```python
from build123d import *

# Parameters (mm, degrees)
CROQUIS1_W              = 240
CROQUIS1_H              = 70
SALIENTE_EXTRUIR1_DEPTH = 5
CROQUIS2_R              = 2.25
CORTAR_EXTRUIR1_DEPTH   = 126.39936204
CROQUIS5_W              = 35
CROQUIS5_H              = 10
CORTAR_EXTRUIR4_DEPTH   = 126.39936204
CROQUIS6_R              = 2.5
CORTAR_EXTRUIR5_DEPTH   = 126.39936204


with BuildPart() as part:
    # Croquis1 → Saliente-Extruir1 (new, symmetric)
    with BuildSketch(Plane(origin=(0, 0, 0), x_dir=(1, 0, 0), z_dir=(0, 1, 0))):
        Rectangle(CROQUIS1_W, CROQUIS1_H)
    extrude(amount=SALIENTE_EXTRUIR1_DEPTH, both=True)

    # Croquis2 → Cortar-Extruir1 (cut, through all)
    with BuildSketch(Plane(origin=(0, 5, 0), x_dir=(1, 0, 0), z_dir=(0, 1, 0))):
        with Locations(Location((-115, 20, 0), (0, 0, 270))):
            Circle(CROQUIS2_R)
        with Locations(Location((-115, -20, 0), (0, 0, 270))):
            Circle(CROQUIS2_R)
        with Locations(Location((115, -20, 0), (0, 0, 90))):
            Circle(CROQUIS2_R)
        with Locations(Location((115, 20, 0), (0, 0, 90))):
            Circle(CROQUIS2_R)
    extrude(amount=-CORTAR_EXTRUIR1_DEPTH, mode=Mode.SUBTRACT)

    # Croquis5 → Cortar-Extruir4 (cut, through all)
    with BuildSketch(Plane(origin=(0, 5, 0), x_dir=(1, 0, 0), z_dir=(0, 1, 0))):
        with Locations((-31.75, 21.46)):
            Rectangle(CROQUIS5_W, CROQUIS5_H)
        with Locations((-31.75, -21.71)):
            Rectangle(CROQUIS5_W, CROQUIS5_H)
        with Locations((31.75, 21.46)):
            Rectangle(CROQUIS5_W, CROQUIS5_H)
        with Locations((31.75, -21.71)):
            Rectangle(CROQUIS5_W, CROQUIS5_H)
    extrude(amount=-CORTAR_EXTRUIR4_DEPTH, mode=Mode.SUBTRACT)

    # Croquis6 → Cortar-Extruir5 (cut, through all)
    with BuildSketch(Plane(origin=(0, 5, 0), x_dir=(1, 0, 0), z_dir=(0, 1, 0))):
        with Locations(Location((71.38, 0, 0), (0, 0, 270))):
            Circle(CROQUIS6_R)
        with Locations(Location((-91.85, 0, 0), (0, 0, 270))):
            Circle(CROQUIS6_R)
    extrude(amount=-CORTAR_EXTRUIR5_DEPTH, mode=Mode.SUBTRACT)


solid = part.part
```
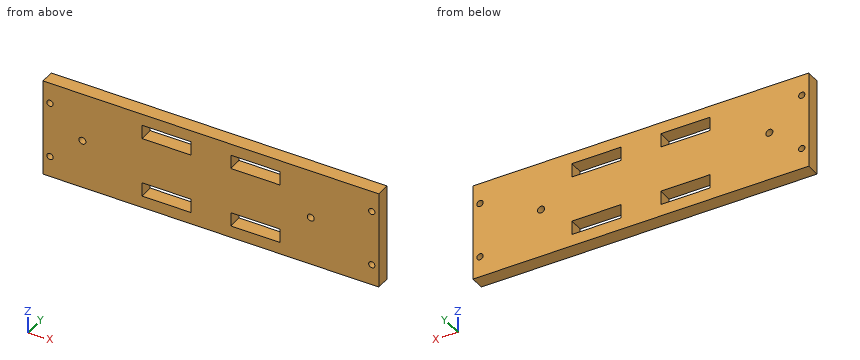
Here's how the part is built. I have some questions about the finished solid (model axes, mm). Coordinates: 2 decimals unless noted, no trailing zeros. Order: outer loops, then holes, each group sorted by start corner. A loop starts at its lowest first (then second) coordinate and runs counter-clockwise, first axis right, second up.
1) Imagine slicing it at B-B on z = 20. List the corners of the cut face in (x, y) for me, and give its area (3 significant figures).
2) Imagine slicing it at C-C on y = -2.5. State how many separate pieces and enclosed holes the cut face has, and give its area (3 significant figures).
3) Imagine slicing it at D-D on x = -91.85. List the corners of the cut face in (y, z) for me, and give its area (3 significant figures).
4) I need wall thicknesses on line 1 (X direction, y = -1, z = 20); line 2 (X direction, y = -1.25, z = 23.5); line 3 (Z direction, x = 115, y = 1). Which ranges of each line are inside material? Lowest first, please.
5) Imagine slicing it at A-A on x = 42. List the corners of the cut face in (y, z) for me.
Response values:
1. outline: (-120, -5) - (-117.25, -5) - (-117.25, 5) - (-120, 5) - close; (-112.75, -5) - (-49.25, -5) - (-49.25, 5) - (-112.75, 5) - close; (-14.25, -5) - (14.25, -5) - (14.25, 5) - (-14.25, 5) - close; (49.25, -5) - (112.75, -5) - (112.75, 5) - (49.25, 5) - close; (117.25, -5) - (120, -5) - (120, 5) - (117.25, 5) - close
1. area: 1,610 mm2
2. separate pieces: 1
2. enclosed holes: 10
2. area: 15,300 mm2
3. outline: (-5, -35) - (5, -35) - (5, -2.5) - (-5, -2.5) - close; (-5, 2.5) - (5, 2.5) - (5, 35) - (-5, 35) - close
3. area: 650 mm2
4. line 1: x = -120 to -117.25, -112.75 to -49.25, -14.25 to 14.25, 49.25 to 112.75, 117.25 to 120
4. line 2: x = -120 to -49.25, -14.25 to 14.25, 49.25 to 120
4. line 3: z = -35 to -22.25, -17.75 to 17.75, 22.25 to 35
5. outline: (-5, -35) - (5, -35) - (5, -26.46) - (-5, -26.46) - close; (-5, -16.46) - (5, -16.46) - (5, 16.71) - (-5, 16.71) - close; (-5, 26.71) - (5, 26.71) - (5, 35) - (-5, 35) - close
